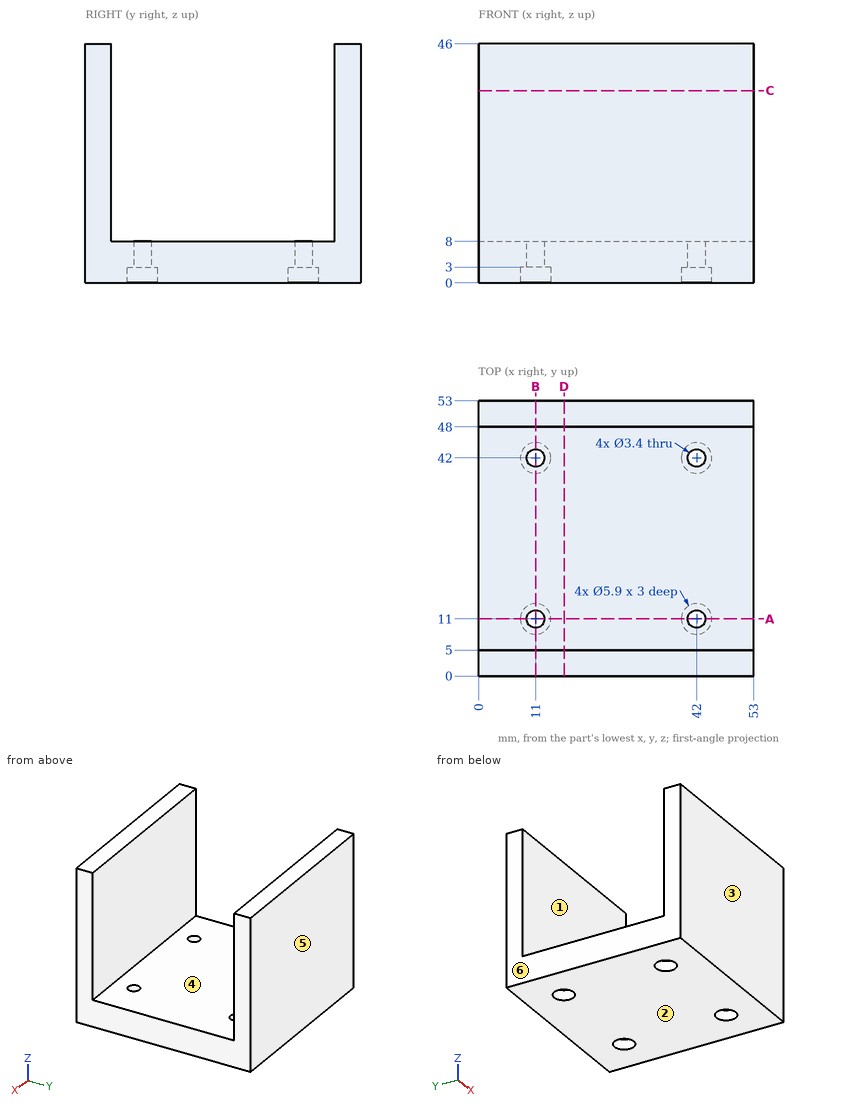
Could you check a few things on this drawing? It's one solid part, dimensions in mm from its lowest x, y, z. A direction names the side the tool comes from. Coordinates: 2 decimals unless noted, no trailing zeros. Write each loop counter-clockwise with the first axis right and the second up, starting at its lowest first coordinate (ties: lowest second). Pieces come first, ordered by that corner, then holes. Notation, with made-up numbers: (57, 52) - (102, 52) arc R31 cw to (102, 89) - close; hole circle Ø3 at (62.5, 16). An arc over 180 degrees is marked (long way). Put each result on its own line as item: value. Start each with the question number.
Q1. Thinking about a two-plate mould opening in Y: for the marked faces 3, 4, 5 and 6, which applies, pulls with the +Y half, pulls with the -Y half, needs draft (parallel to the pull), parting line crosses it, or undercut?
Q2. I want a section at C-C on z = 37. Write out the boundary of the cut face in (x, y), plus the area to 3 significant figures.
Q3. Please list where these lines run through material, in increasing order: L1, parallel to Y at x = 42, z = 1; L2, parallel to Y at x = 42, z = 6; L3, parallel to Y at x = 21.5, z = 11.
Q4. Which directions (+Z, -Z, +X, -X, +Y, -Y) give clear straight access to the entire face, cutting with the end or side of a thin tool? Please do the marked faces 1 and 2.
Q5. I want a section at B-B on x = 11. Write out the boundary of the cut face in (y, z), plus the area to 3 significant figures.
Q6. I want a section at D-D on x = 16.5. Write out the boundary of the cut face in (y, z), plus the area to 3 significant figures.
Q7. I want a section at A-A on y = 11. Write out the boundary of the cut face in (x, z), plus the area to 3 significant figures.
Q8. I'm going to push flat-ended pins straight in: P1, Ø6, axis at x = 41.5, y = 6.5, coming from the -Z side; P2, Ø3, axis at x = 42, y = 42, coming from the +Z side; P3, Ø4.5, axis at x = 11, y = 42, coming from the +Z side; P4, Ø4.5, axis at x = 11, y = 42, coming from the -Z side. Where does each tip first touch, or does it pass through?
Checks:
1. face 3: pulls with the -Y half
1. face 4: undercut
1. face 5: pulls with the +Y half
1. face 6: needs draft
2. outline: (0, 0) - (53, 0) - (53, 5) - (0, 5) - close; (0, 48) - (53, 48) - (53, 53) - (0, 53) - close
2. area: 530 mm²
3. L1: 0 to 8.05, 13.95 to 39.05, 44.95 to 53
3. L2: 0 to 9.3, 12.7 to 40.3, 43.7 to 53
3. L3: 0 to 5, 48 to 53
4. face 1: +Z, +X, -X
4. face 2: -Z, +X, -X, +Y, -Y
5. outline: (0, 0) - (8.05, 0) - (8.05, 3) - (9.3, 3) - (9.3, 8) - (5, 8) - (5, 46) - (0, 46) - close; (12.7, 3) - (13.95, 3) - (13.95, 0) - (39.05, 0) - (39.05, 3) - (40.3, 3) - (40.3, 8) - (12.7, 8) - close; (43.7, 3) - (44.95, 3) - (44.95, 0) - (53, 0) - (53, 46) - (48, 46) - (48, 8) - (43.7, 8) - close
5. area: 735 mm²
6. outline: (0, 0) - (53, 0) - (53, 46) - (48, 46) - (48, 8) - (5, 8) - (5, 46) - (0, 46) - close
6. area: 804 mm²
7. outline: (0, 0) - (8.05, 0) - (8.05, 3) - (9.3, 3) - (9.3, 8) - (0, 8) - close; (12.7, 3) - (13.95, 3) - (13.95, 0) - (39.05, 0) - (39.05, 3) - (40.3, 3) - (40.3, 8) - (12.7, 8) - close; (43.7, 3) - (44.95, 3) - (44.95, 0) - (53, 0) - (53, 8) - (43.7, 8) - close
7. area: 355 mm²
8. P1: z = 0
8. P2: through
8. P3: z = 8
8. P4: z = 3
